Read the model definition and answer for the solid it produces. Units are mm, in the model's axes. Face numbers are marked on the shaded views. A direction names the side the tool comes from. Round coordinates to 2 decimals unless told otherwise and drop trailing zeros. Write each loop counter-clockwise with the first axis right and the second up, starting at its lowest first coordinate (ties: lowest second). Pieces come first, ordered by that corner, then holes. Notation, with made-up numbers: (11.5, -26) -> (60.5, -26) arc R9 ccw to (60.5, -11) -> close; hole circle Ø1 at (10, 51). An arc over 180 degrees is marked (long way). Return JSON: item names as keys, results as strings. Group by question number.
(1) The mould has two halves that part along X. Classify the marked faces 3, 4 and 5: released by +X, released by -X, zero draft, split by the parting line, or undercut.
(2) For the marked faces 1 and 2, determine the directions among +Z, -Z, +X, -X, +Y, -Y from which every point of the face is accessible in a straight line to the end or side of a thin tool.
(3) Straight lines are drawn through the part: line 1 (Z direction, x = 3, y = 56); line 2 (X direction, y = 96.5, z = 22). For each, find the intervals that lie inside material, in ascending order.
(4) A cutting plane is placed at A-A on z = 0.5. Give the vertices of the cut face in (x, y), then the cut area to 3 significant figures.
(5) A cutting plane is placed at C-C on y = 112.5. Give the vertices of the cut face in (x, z), then the cut area to 3 significant figures.
(6) A cutting plane is placed at B-B on x = -12. Give the vertices of the cut face in (y, z), then the cut area to 3 significant figures.
Autodesk Inventor part; units mm, degrees
ref_plane "РабПлоскость1" through (0, 104, 0) normal (0, 1, 0) x (1, 0, 0)
ref_plane "YZ Plane" through (0, 0, 0) normal (1, 0, 0) x (0, 1, 0)
ref_plane "XZ Plane" through (0, 0, 0) normal (0, 1, 0) x (-1, 0, 0)
sketch "Эскиз1" plane through (0, 0, 0) normal (0, 1, 0) x (-1, 0, 0)
  line L0 (-25, -20.5) -> (-25, 20.5)
  line L1 (-20.5, 25) -> (20.5, 25)
  line L2 (25, 20.5) -> (25, -20.5)
  line L3 (20.5, -25) -> (-20.5, -25)
  arc A0 (-25, -20.5) -> (-20.5, -25) centre (-20.5, -20.5) ccw
  arc A1 (-20.5, 25) -> (-25, 20.5) centre (-20.5, 20.5) ccw
  arc A2 (25, 20.5) -> (20.5, 25) centre (20.5, 20.5) ccw
  arc A3 (20.5, -25) -> (25, -20.5) centre (20.5, -20.5) ccw
  arc A4 (-20.5, 22) -> (-22, 20.5) centre (-20.5, 20.5) ccw
  line L4 (-20.5, 22) -> (20.5, 22)
  arc A5 (22, 20.5) -> (20.5, 22) centre (20.5, 20.5) ccw
  line L5 (22, 20.5) -> (22, -20.5)
  arc A6 (20.5, -22) -> (22, -20.5) centre (20.5, -20.5) ccw
  line L6 (20.5, -22) -> (-20.5, -22)
  arc A7 (-22, -20.5) -> (-20.5, -22) centre (-20.5, -20.5) ccw
  line L7 (-22, -20.5) -> (-22, 20.5)
  line L8 (0, 36.3048) -> (0, -36.3048) construction
  line L9 (-36.3048, 0) -> (36.3048, 0) construction
  arc A8 (20.5, -26) -> (26, -20.5) centre (20.5, -20.5) ccw
  line L10 (20.5, -26) -> (-20.5, -26)
  arc A9 (-26, -20.5) -> (-20.5, -26) centre (-20.5, -20.5) ccw
  line L11 (-26, -20.5) -> (-26, 20.5)
  arc A10 (-20.5, 26) -> (-26, 20.5) centre (-20.5, 20.5) ccw
  line L12 (-20.5, 26) -> (20.5, 26)
  arc A11 (26, 20.5) -> (20.5, 26) centre (20.5, 20.5) ccw
  line L13 (26, 20.5) -> (26, -20.5)
  arc A12 (20.5, -24) -> (24, -20.5) centre (20.5, -20.5) ccw
  line L14 (20.5, -24) -> (-20.5, -24)
  arc A13 (-24, -20.5) -> (-20.5, -24) centre (-20.5, -20.5) ccw
  line L15 (-24, -20.5) -> (-24, 20.5)
  arc A14 (-20.5, 24) -> (-24, 20.5) centre (-20.5, 20.5) ccw
  line L16 (-20.5, 24) -> (20.5, 24)
  arc A15 (24, 20.5) -> (20.5, 24) centre (20.5, 20.5) ccw
  line L17 (24, 20.5) -> (24, -20.5)
  point P0 (0, 0)
  dimension "d0" = 4.5
  dimension "d1" = 50
  dimension "d2" = 50
  dimension "d3" = 3
  dimension "d4" = 25
  dimension "d5" = 25
  dimension "d10" = 1
  dimension "d13" = 1
extrude "Выдавливание1" add sketch "Эскиз1" along normal blind 129 contours L0 A1 L1 A2 L2 A3 L3 A0
ref_plane "РабПлоскость1" through (0, 104, 0) normal (0, 1, 0) x (1, 0, 0)
split_face "Разделение1"
equation "\"d0\" = d6"
equation "\"d1\" = d7"
equation "\"d2\" = d8"
equation "\"d3\" = d9"
equation "\"d4\" = 0.5 * d1"
equation "\"d5\" = 0.5 * d2"
equation "\"d6\" = 1.5 * d9"
equation "\"d7\" = 50"
equation "\"d8\" = 50"
equation "\"d9\" = 3"
properties part number "Fiberglass_isolation" material "Стекловолоконная обертывающая изоляция"
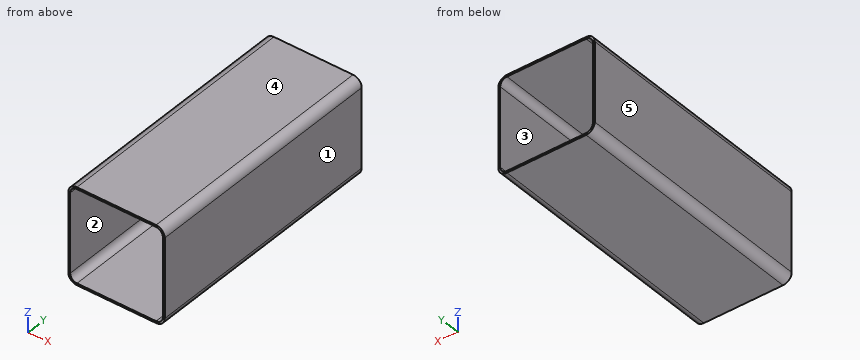
Checks:
{
 "1": {"face 3": "undercut", "face 4": "zero draft", "face 5": "released by -X"},
 "2": {"face 1": "+Z, -Z, +X, +Y, -Y", "face 2": "+Y, -Y"},
 "3": {"line 1": "z = -25 to -24, 24 to 25", "line 2": "x = -24.74 to -23.66, 23.66 to 24.74"},
 "4": {"outline": "(-25, 0) -> (-24, 0) -> (-24, 129) -> (-25, 129) -> close; (24, 0) -> (25, 0) -> (25, 129) -> (24, 129) -> close", "area": "258 mm^2"},
 "5": {"outline": "(-25, -20.5) arc R4.5 ccw to (-20.5, -25) -> (20.5, -25) arc R4.5 ccw to (25, -20.5) -> (25, 20.5) arc R4.5 ccw to (20.5, 25) -> (-20.5, 25) arc R4.5 ccw to (-25, 20.5) -> close; hole (-24, -20.5) arc R3.5 ccw to (-20.5, -24) -> (20.5, -24) arc R3.5 ccw to (24, -20.5) -> (24, 20.5) arc R3.5 ccw to (20.5, 24) -> (-20.5, 24) arc R3.5 ccw to (-24, 20.5) -> close", "area": "189 mm^2"},
 "6": {"outline": "(0, -25) -> (129, -25) -> (129, -24) -> (0, -24) -> close; (0, 24) -> (129, 24) -> (129, 25) -> (0, 25) -> close", "area": "258 mm^2"}
}
